```python
from build123d import *

# Parameters (mm, degrees)
SKETCH1_R                 = 5
SKETCH1_R_2               = 2.55
BOSS_EXTRUDE1_DEPTH       = 5
FILLET1_R                 = 0.5
F_2_5MM_DOWEL_HOLE1_D     = 2.4
F_2_5MM_DOWEL_HOLE1_DEPTH = 5
F_2_5MM_DOWEL_HOLE1_TIP   = 0.721032743


with BuildPart() as part:
    # Sketch1 → Boss-Extrude1 (new body)
    with BuildSketch(Plane(origin=(0, 0, 0), x_dir=(1, 0, 0), z_dir=(0, 1, 0))):
        with Locations(Location((0, 0, 0), (0, 0, 270))):
            Circle(SKETCH1_R)
        with Locations(Location((0, 0, 0), (0, 0, 270))):
            Circle(SKETCH1_R_2, mode=Mode.SUBTRACT)
    extrude(amount=BOSS_EXTRUDE1_DEPTH)

    # Fillet1
    fillet1_edges = [part.edges().sort_by_distance(p)[0] for p in [
        (0, 0, -5),
        (0, 5, -5),
        (0, 0, -2.55),
        (0, 5, -2.55),
    ]]
    fillet(fillet1_edges, radius=FILLET1_R)

    # Ø2.5mm Dowel Hole1
    with Locations(Plane(origin=(5, 2.491746689, 0), x_dir=(0, 0, 1), z_dir=(1, 0, 0))):
        with Locations((0, 0)):
            Hole(F_2_5MM_DOWEL_HOLE1_D / 2, depth=F_2_5MM_DOWEL_HOLE1_DEPTH)
            with Locations((0, 0, -(F_2_5MM_DOWEL_HOLE1_DEPTH + F_2_5MM_DOWEL_HOLE1_TIP / 2))):  # 118° drill point
                Cone(0, F_2_5MM_DOWEL_HOLE1_D / 2, F_2_5MM_DOWEL_HOLE1_TIP, mode=Mode.SUBTRACT)


solid = part.part
```
Geometry: final body of the model. Coordinates: model frame, mm. A direction names the side the tool comes from. Round coordinates to 2 decimals unless told otherwise and drop trailing zeros. Order: outer loops, then holes, each group sorted by start corner. A loop starts at its lowest first (then second) coordinate and runs counter-clockwise, first axis right, second up. Notation, with made-up numbers: M 12.25,-0.75 L 39.25,-0.75 A27 cw 39.25,32.25 Z; hole C 20.5,-7 d11. An arc over 180 degrees is marked long. One line per item, written item: value.
(1) Reachability of faces 1 (the cylindrical face through (-4.88, 2.47, -1.08)), 2 (the cylindrical face through (3.61, 3.56, -0.55)) from +Z, -Z, +X, -X, +Y, -Y: full face, straight path, thin tool, end or side. Return the list, or none.
Result sheet:
face 1: +Y, -Y
face 2: +X
(2) Pin query (flat end, axial travel): P1, Ø3, axis at x = 0, z = 0, coming from the -Y side (1 decimal); P2, Ø1.5, axis at x = 3.5, y = 4, coming from the +Z side; P3, Ø1, axis at y = 3, z = -2, coming from the -X side; P4, Ø3, axis at x = -2, y = 4, coming from the +Z side. Return the tip coordinate at first contact, or that it passes through.
Result sheet:
P1: through
P2: z = 4.18
P3: x = -4.77
P4: z = 4.97
(3) Cut plane D-D (y = 1.8). Return the cut outline in (x, z).
Result sheet:
outline: M 2.35,-0.98 A2.55 cw long 2.35,0.98 L 4.9,0.98 A5 ccw long 4.9,-0.98 Z
(4) Cut plane A-A (x = 0). Return the cut outline in (y, z), and give its area (3 significant figures).
Result sheet:
outline: M 0,-4.5 A0.5 ccw 0.5,-5 L 4.5,-5 A0.5 ccw 5,-4.5 L 5,-3.05 A0.5 ccw 4.5,-2.55 L 0.5,-2.55 A0.5 ccw 0,-3.05 Z; M 0,3.05 A0.5 ccw 0.5,2.55 L 4.5,2.55 A0.5 ccw 5,3.05 L 5,4.5 A0.5 ccw 4.5,5 L 0.5,5 A0.5 ccw 0,4.5 Z
area: 24.1 mm2
(5) Cut plane C-C (z = 1). Give the number of separate pieces and of enclosed holes in the cut face, and give its area (3 significant figures).
Result sheet:
separate pieces: 3
enclosed holes: 0
area: 21.7 mm2
(6) Line query: probe 1 along Y at (x, z) = (3.65, 0); probe 2 along X at (y, z) = (1.6, 0); probe 3 along Z at (x, y) = (0.25, 1.1). Output: solid intervals per line, ascending. Write a range as [from, to].
Result sheet:
probe 1: [0, 1.29], [3.69, 5]
probe 2: [-5, -2.55]
probe 3: [-4.99, -2.54], [2.54, 4.99]
(7) Cut plane B-B (y = 4.35). Return the cut outline in (x, z).
Result sheet:
outline: C 0,0 d10; hole C 0,0 d5.1
